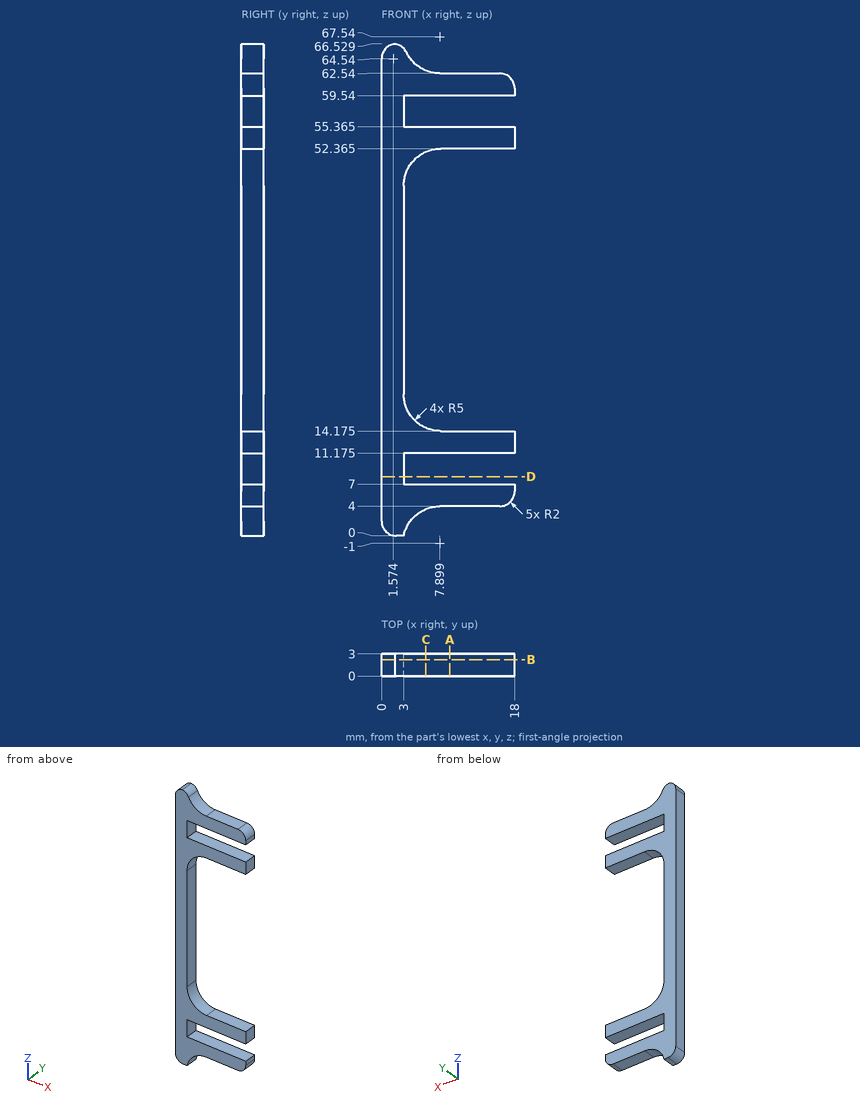
The figure shows three views and two pictorial views of one solid part (mm, origin at its lowest corner). Answer the questions. Coordinates: 2 decimals unless noted, no trailing zeros. Loops run counter-clockwise (first coordinate to the right, second up) from the corner with the lowest first, then second, coordinate; pieces in that order, holes last. Notation, with made-up numbers: M 61,71 L 113,71 A35 ccw 113,107 Z; hole C -30.5,-16 d2. An arc over 180 degrees is marked long. Use CSV: the item, a comma, the result in double quotes. Start each with the question number.
(1) Consider line 1 (Z direction, x = 15.25, y = 1) (1 decimal); line 2 (Z direction, x = 6.75, y = 0.75) (1 decimal); line 3 (X direction, y = 1.45, z = 25). Determine where each line is inside the solid, lowest interval first.
(2) Find section B-B, the plane y = 2.2. Give the vertices of the cut face in (x, z) (1 decimal).
(3) Find section A-A, the plane x = 9.25. Give the vertices of the cut face in (y, z) (1 decimal), then the cut area to 3 significant figures.
(4) Find section C-C, the plane x = 6. Give the vertices of the cut face in (y, z) (1 decimal).
(5) Given pin 1 Ø1.5 at (x, y) = (11.5, 2) entering from +Z; pin 2 Ø1.5 at (x, y) = (8, 2) entering from -Z; pin 3 Ø0.9 at (x, y) = (8, 1) entering from +Z, each flat-ended and moving along its own axis, determine where each tip first touches the part or whether it passes through.
(6) Find section D-D, the plane z = 8. Give the vertices of the cut face in (x, y).
Recorded:
1,line 1,"z = 4 to 7, 11.2 to 14.2, 52.4 to 55.4, 59.5 to 62.5"
1,line 2,"z = 3.9 to 7, 11.2 to 14.3, 52.2 to 55.4, 59.5 to 62.7"
1,line 3,"x = 0 to 3"
2,outline,"M 0,2 A2 ccw 2,0 L 3,0 A5 cw 7.9,4 L 16,4 A2 ccw 18,6 L 18,7 L 3,7 L 3,11.2 L 18,11.2 L 18,14.2 L 8,14.2 A5 cw 3,19.2 L 3,47.4 A5 cw 8,52.4 L 18,52.4 L 18,55.4 L 3,55.4 L 3,59.5 L 18,59.5 L 18,60.5 A2 ccw 16,62.5 L 7.9,62.5 A5 cw 3.4,65.4 A2 ccw 1.8,66.5 A2 ccw 0,64.5 Z"
3,outline,"M 0,4 L 3,4 L 3,7 L 0,7 Z; M 0,11.2 L 3,11.2 L 3,14.2 L 0,14.2 Z; M 0,52.4 L 3,52.4 L 3,55.4 L 0,55.4 Z; M 0,59.5 L 3,59.5 L 3,62.5 L 0,62.5 Z"
3,area,"36.0 mm^2"
4,outline,"M 0,3.6 L 3,3.6 L 3,7 L 0,7 Z; M 0,11.2 L 3,11.2 L 3,14.6 L 0,14.6 Z; M 0,51.9 L 3,51.9 L 3,55.4 L 0,55.4 Z; M 0,59.5 L 3,59.5 L 3,62.9 L 0,62.9 Z"
5,pin 1,"stops at z = 62.54"
5,pin 2,"stops at z = 3.96"
5,pin 3,"stops at z = 62.55"
6,outline,"M 0,0 L 3,0 L 3,3 L 0,3 Z"
